Can you work these out from the drawing? Everything is in mm from the part's minimum corner. A direction names the side the tool comes from. Give positions to 0.01 mm unless a question says otherwise; leave off trailing zeros. Order: outer loops, then holes, each group sorted by start corner. A loop starts at its lowest first (then second) coordinate and runs counter-clockwise, first axis right, second up. Notation, with made-up numbers: (61.25, -10.5) -> (94.25, -10.5) arc R24 cw to (94.25, 24.5) -> close; hole circle Ø6 at (24, 28). An arc over 180 degrees is marked (long way). One line per item, written item: value.
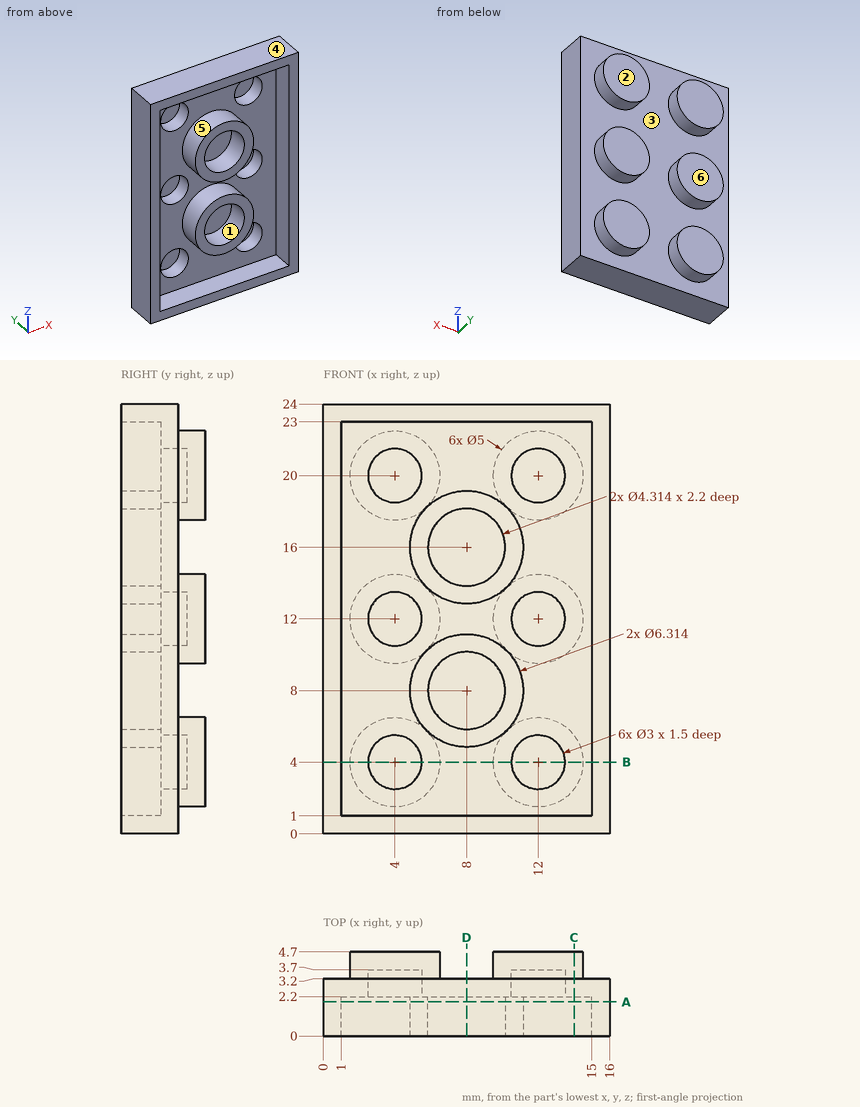
1) Suppose I cut it at A-A, the plane y = 1.9. Write out the boundary of the cut face in (x, z).
Answer below:
outline: (0, 0) -> (16, 0) -> (16, 24) -> (0, 24) -> close; circle Ø6.31 at (8, 8); circle Ø6.31 at (8, 16); hole (1, 1) -> (15, 1) -> (15, 23) -> (1, 23) -> close; hole circle Ø4.31 at (8, 8); hole circle Ø4.31 at (8, 16)
2) If I drill on line 1 along Z through (x, y) = (14, 4.25); line 2 along X through (y, z) = (3.05, 4); line 3 along Z through (x, y) = (4, 2.95), over which ranges is the centre line in solid material (lowest first)?
Answer below:
line 1: z = 2.5 to 5.5, 10.5 to 13.5, 18.5 to 21.5
line 2: x = 0 to 2.5, 5.5 to 10.5, 13.5 to 16
line 3: z = 0 to 2.5, 5.5 to 10.5, 13.5 to 18.5, 21.5 to 24
3) For P1, Ø1.3, axis at x = 8.5, z = 7.5, coming from the -Y side; P2, Ø1.5, axis at x = 8.5, y = 4, coming from the +Z side; P3, Ø1.5, axis at x = 4, z = 19.5, coming from the -Y side, each with a flat end and sliding along its axis, tell me the tip position at first contact or that it passes through.
Answer below:
P1: stops at y = 2.2
P2: passes through
P3: stops at y = 3.7
4) Suppose I cut it at B-B, the plane z = 4. Write out the boundary of the cut face in (x, y), then the cut area to 3 significant figures.
Answer below:
outline: (0, 0) -> (1, 0) -> (1, 2.2) -> (2.5, 2.2) -> (2.5, 3.7) -> (5.5, 3.7) -> (5.5, 2.2) -> (10.5, 2.2) -> (10.5, 3.7) -> (13.5, 3.7) -> (13.5, 2.2) -> (15, 2.2) -> (15, 0) -> (16, 0) -> (16, 3.2) -> (14.5, 3.2) -> (14.5, 4.7) -> (9.5, 4.7) -> (9.5, 3.2) -> (6.5, 3.2) -> (6.5, 4.7) -> (1.5, 4.7) -> (1.5, 3.2) -> (0, 3.2) -> close
area: 26.4 mm2
5) We'd pull the mould along Z, two halves only. Please class the marked faces 1, 2, 3 and 4: +Z half, -Z half, draft (parallel to the pull), parting line (faces both ways), or undercut.
Answer below:
face 1: undercut
face 2: draft
face 3: undercut
face 4: +Z half
6) Suppose I cut it at C-C, the plane x = 14. Write out the boundary of the cut face in (y, z).
Answer below:
outline: (0, 0) -> (3.2, 0) -> (3.2, 2.5) -> (4.7, 2.5) -> (4.7, 5.5) -> (3.2, 5.5) -> (3.2, 10.5) -> (4.7, 10.5) -> (4.7, 13.5) -> (3.2, 13.5) -> (3.2, 18.5) -> (4.7, 18.5) -> (4.7, 21.5) -> (3.2, 21.5) -> (3.2, 24) -> (0, 24) -> (0, 23) -> (2.2, 23) -> (2.2, 1) -> (0, 1) -> close
7) For the marked faces 5 and 6, which set-ups out of +Z, -Z, +X, -X, +Y, -Y let a thin tool reach every point of the face, with its end or its side?
Answer below:
face 5: -Y
face 6: +Z, -Z, +X, -X, +Y
8) Suppose I cut it at D-D, the plane x = 8. Write out the boundary of the cut face in (y, z).
Answer below:
outline: (0, 0) -> (3.2, 0) -> (3.2, 24) -> (0, 24) -> (0, 23) -> (2.2, 23) -> (2.2, 19.16) -> (0, 19.16) -> (0, 18.16) -> (2.2, 18.16) -> (2.2, 13.84) -> (0, 13.84) -> (0, 12.84) -> (2.2, 12.84) -> (2.2, 11.16) -> (0, 11.16) -> (0, 10.16) -> (2.2, 10.16) -> (2.2, 5.84) -> (0, 5.84) -> (0, 4.84) -> (2.2, 4.84) -> (2.2, 1) -> (0, 1) -> close
